Geometry check sheet. Reference: the model listing, model coordinates, mm. Coordinates: 2 decimals unless noted, no trailing zeros. Loops run counter-clockwise (first coordinate to the right, second up) from the corner with the lowest first, then second, coordinate; pieces in that order, holes last.
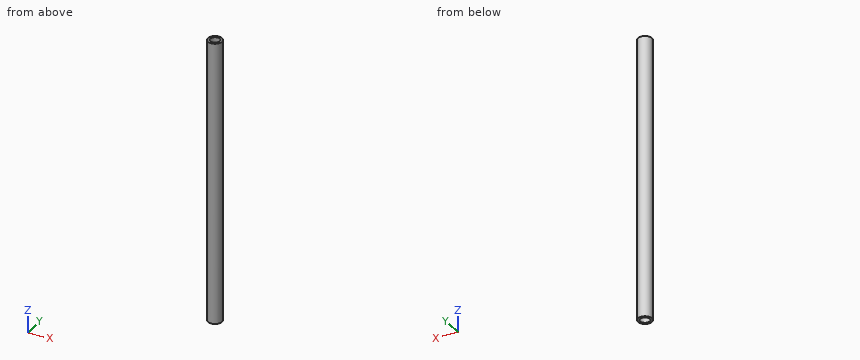
Autodesk Inventor part; units mm, degrees
ref_plane "YZ Plane" through (0, 0, 0) normal (1, 0, 0) x (0, 1, 0)
ref_plane "XZ Plane" through (0, 0, 0) normal (0, 1, 0) x (-1, 0, 0)
ref_plane "XY Plane" through (0, 0, 0) normal (0, 0, 1) x (1, 0, 0)
sketch "Sketch1" plane through (0, 0, 0) normal (0, 0, 1) x (1, 0, 0)
  circle A0 centre (0, 0) radius 2
  circle A1 centre (0, 0) radius 1.375
  circle A2 centre (0, 0) radius 2.875
  circle A3 centre (0, 0) radius 2.25
  dimension "d0" = 4
  dimension "d1" = 2.75
  dimension "d2" = 5.75
  dimension "d3" = 4.5
extrude "Extrusion1" add sketch "Sketch1" along normal blind 81 contours A0 | A1
sketch "Sketch2" plane through (0, 0, 81) normal (0, 0, 1) x (1, 0, 0)
  circle A0 centre (0, 0) radius 1.375
  dimension "d9" = 2.75
extrude "Extrusion3" cut sketch "Sketch2" against normal blind 6
extrude "Extrusion4" cut sketch "Sketch1" along normal blind 6 contours A1
properties part number "Schanier pin"
(1) Scan lines: L1, parallel to Y at x = 0, z = 2.45 (3 decimals); L2, parallel to X at y = 0.1, z = 44.5; L3, parallel to Z at x = 0, y = -0.7. Record each from-to range of solid material in increasing order.
Findings:
L1: y = -2 to -1.375, 1.375 to 2
L2: x = -2 to 2
L3: z = 6 to 75
(2) Gauge pin test, flat ends, axial feed: pin 1 Ø1 at (y, z) = (-1, 54) entering from -X; pin 2 Ø2 at (x, y) = (-0.5, 0.5) entering from -Z. Record the tip position at first contact, or that the pin passes through.
Findings:
pin 1: stops at x = -1.94
pin 2: stops at z = 0
(3) Sectioned sample at C-C on z = 41. Record the cut outline in (x, y).
Findings:
outline: circle Ø4 at (0, 0)
(4) Sectioned sample at A-A on y = 0. Record the cut outline in (x, z) (3 decimals), and give its area (3 significant figures).
Findings:
outline: (-2, 0) - (-1.375, 0) - (-1.375, 6) - (1.375, 6) - (1.375, 0) - (2, 0) - (2, 81) - (1.375, 81) - (1.375, 75) - (-1.375, 75) - (-1.375, 81) - (-2, 81) - close
area: 291 mm2
